For this review, take the finished solid that the model builds, in its own axes (mm). Round coordinates to 2 decimals unless told otherwise and drop trailing zeros. Write each loop counter-clockwise with the first axis right and the second up, starting at its lowest first coordinate (ties: lowest second). Pieces come first, ordered by that corner, then holes. Notation, with made-up numbers: (78, 77) -> (86, 77) arc R26 ccw to (86, 108) -> close; hole circle Ø9 at (77, 79.5). An arc over 180 degrees is marked (long way). Write item = value, one per line. Start each with the question number.
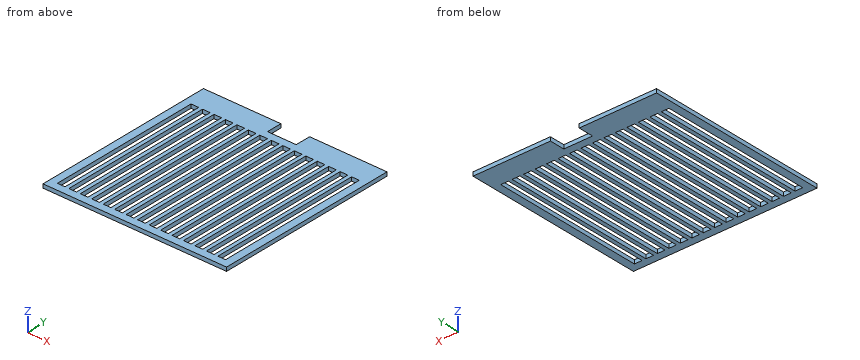
```python
from build123d import *

# Parameters (mm, degrees)
SKETCH1_W             = 96
SKETCH1_H             = 96
BOSS_EXTRUDE2_DEPTH   = 2
FINGER_OPENING_HOLE_W = 15
FINGER_OPENING_HOLE_H = 8
OPENING_HOLE_DEPTH    = 2
AIRFLOW_W             = 4
AIRFLOW_H             = 80
AIR_FLOW_DEPTH        = 2


with BuildPart() as part:
    # Sketch1 → Boss-Extrude2 (new body)
    with BuildSketch(Plane.XY):
        with Locations((48, 48)):
            Rectangle(SKETCH1_W, SKETCH1_H)
    extrude(amount=BOSS_EXTRUDE2_DEPTH)

    # Finger Opening Hole → Opening Hole (cut)
    with BuildSketch(Plane.XY.offset(2)):
        with Locations((48, 92)):
            Rectangle(FINGER_OPENING_HOLE_W, FINGER_OPENING_HOLE_H)
    extrude(amount=-OPENING_HOLE_DEPTH, mode=Mode.SUBTRACT)

    # Airflow → Air Flow (cut)
    with BuildSketch(Plane.XY.offset(2)):
        with Locations((12, 44)):
            Rectangle(AIRFLOW_W, AIRFLOW_H)
        with Locations((6, 44)):
            Rectangle(AIRFLOW_W, AIRFLOW_H)
        with Locations((18, 44)):
            Rectangle(AIRFLOW_W, AIRFLOW_H)
        with Locations((24, 44)):
            Rectangle(AIRFLOW_W, AIRFLOW_H)
        with Locations((30, 44)):
            Rectangle(AIRFLOW_W, AIRFLOW_H)
        with Locations((36, 44)):
            Rectangle(AIRFLOW_W, AIRFLOW_H)
        with Locations((42, 44)):
            Rectangle(AIRFLOW_W, AIRFLOW_H)
        with Locations((48, 44)):
            Rectangle(AIRFLOW_W, AIRFLOW_H)
        with Locations((54, 44)):
            Rectangle(AIRFLOW_W, AIRFLOW_H)
        with Locations((60, 44)):
            Rectangle(AIRFLOW_W, AIRFLOW_H)
        with Locations((66, 44)):
            Rectangle(AIRFLOW_W, AIRFLOW_H)
        with Locations((72, 44)):
            Rectangle(AIRFLOW_W, AIRFLOW_H)
        with Locations((78, 44)):
            Rectangle(AIRFLOW_W, AIRFLOW_H)
        with Locations((84, 44)):
            Rectangle(AIRFLOW_W, AIRFLOW_H)
        with Locations((90, 44)):
            Rectangle(AIRFLOW_W, AIRFLOW_H)
    extrude(amount=-AIR_FLOW_DEPTH, mode=Mode.SUBTRACT)


solid = part.part
```
1. Consider section A-A, the plane x = 72. Give the boundary of the cut face in (y, z), then the cut area to 3 significant figures.
2. Wall thickness on L1, parallel to Y at x = 6, z = 1.3: over which ranges is the line inside the solid? List them lowest first. Write a range as from..to.
3. Consider section B-B, the plane z = 0.5. Give the number of separate pieces and of enclosed holes in the cut face, then the cut area to 3 significant figures.
Outcome:
q1.outline = (0, 0) -> (4, 0) -> (4, 2) -> (0, 2) -> close; (84, 0) -> (96, 0) -> (96, 2) -> (84, 2) -> close
q1.area = 32.0 mm2
q2.L1 = 0..4, 84..96
q3.separate_pieces = 1
q3.enclosed_holes = 15
q3.area = 4,300 mm2
